Autodesk Fusion 360 part; units mm, degrees
sketch "Sketch1" plane through (0, 0, 0) normal (0, 0, 1) x (1, 0, 0)
  circle A0 centre (0, 0) radius 4
  circle A1 centre (0, 0) radius 1.5
  dimension "d1" = 8
  dimension "d2" = 3
extrude "Extrude1" add sketch "Sketch1" along normal blind 4
sketch "Sketch2" plane through (0, 0, 4) normal (0, 0, 1) x (-1, 0, 0)
  circle A0 centre (0, 0) radius 1.5
  circle A1 centre (0, 0) radius 4
  circle A2 centre (0, 0) radius 3.4
  circle A3 centre (0, 0) radius 2.1
  dimension "d5" = -0.6
  dimension "d6" = 0.6
extrude "Extrude2" cut sketch "Sketch2" against normal blind 0.3 contours A2
sketch "Sketch3" plane through (0, 0, 0) normal (0, 0, -1) x (1, 0, 0)
  circle A0 centre (0, 0) radius 1.5
  circle A1 centre (0, 0) radius 4
  circle A2 centre (0, 0) radius 3.4
  circle A3 centre (0, 0) radius 2.1
  dimension "d9" = -0.6
  dimension "d10" = 0.6
extrude "Extrude3" cut sketch "Sketch3" against normal blind 0.3 contours A2
Part model, mm, in its own coordinate system. A direction names the side the tool comes from. Round coordinates to 2 decimals unless told otherwise and drop trailing zeros. Loops run counter-clockwise (first coordinate to the right, second up) from the corner with the lowest first, then second, coordinate; pieces in that order, holes last.
Item 1: Drill centre lines: line 1 (Y direction, x = 0, z = 3.8); line 2 (X direction, y = -1.75, z = 3.85); line 3 (Y direction, x = 0, z = 2.95). Where is each one in solid material? Low to high.
Item 2: Mould opens along Y. For faces 1 (the face through (-0.867, 3.905, 1.972)), 2 (the face through (1.4, -0.9, 0)), 3 (the face through (-0.7, 2.2, 3.7)) say: +Y half, -Y half, draft (parallel to the pull), parting line (faces both ways), or undercut.
Item 3: Cut at D-D, the plane y = 1.75. Give the cut face in (x, z), then the cut area to 3 significant figures.
Item 4: Drop flat-ended pins along their axis: P1, Ø1, axis at x = 1.5, z = 1, coming from the -Y side; P2, Ø1.5, axis at x = 0, y = 2.5, coming from the +Z side. Give the stop position or say it passes through.
Item 5: Cut at A-A, the plane y = 0. Give the cut face in (x, z), then the cut area to 3 significant figures.
Item 6: Cut at C-C, the plane z = 3. Give the cut face in (x, y).
Item 7: 3-axis set-ups, long thin cutter, end or side, ignore diameter. For faces 4 (the face through (-1.5, -0.07, 1.97)), 5 (the face through (0.7, 2.2, 0.3)): which of +Z, -Z, +X, -X, +Y, -Y reach the whole face in a straight line?
A:
1. line 1: y = -4 to -3.4, -2.1 to -1.5, 1.5 to 2.1, 3.4 to 4
1. line 2: x = -3.6 to -2.92, -1.16 to 1.16, 2.92 to 3.6
1. line 3: y = -4 to -1.5, 1.5 to 4
2. face 1: parting line
2. face 2: draft
2. face 3: undercut
3. outline: (-3.6, 0) - (-2.92, 0) - (-2.92, 0.3) - (-1.16, 0.3) - (-1.16, 0) - (1.16, 0) - (1.16, 0.3) - (2.92, 0.3) - (2.92, 0) - (3.6, 0) - (3.6, 4) - (2.92, 4) - (2.92, 3.7) - (1.16, 3.7) - (1.16, 4) - (-1.16, 4) - (-1.16, 3.7) - (-2.92, 3.7) - (-2.92, 4) - (-3.6, 4) - close
3. area: 26.7 mm2
4. P1: stops at y = -3.87
4. P2: stops at z = 4
5. outline: (-4, 0) - (-3.4, 0) - (-3.4, 0.3) - (-2.1, 0.3) - (-2.1, 0) - (-1.5, 0) - (-1.5, 4) - (-2.1, 4) - (-2.1, 3.7) - (-3.4, 3.7) - (-3.4, 4) - (-4, 4) - close; (1.5, 0) - (2.1, 0) - (2.1, 0.3) - (3.4, 0.3) - (3.4, 0) - (4, 0) - (4, 4) - (3.4, 4) - (3.4, 3.7) - (2.1, 3.7) - (2.1, 4) - (1.5, 4) - close
5. area: 18.4 mm2
6. outline: circle Ø8 at (0, 0); hole circle Ø3 at (0, 0)
7. face 4: +Z, -Z
7. face 5: -Z
